Can you work these out from the model? Positions are in its coordinate system, mm. A direction names the side the tool comes from. Give positions to 0.01 mm unless a question says otherwise; leave off trailing zeros. Order: outer loops, then holes, each group sorted by start corner. A loop starts at its lowest first (then second) coordinate and runs counter-clockwise, first axis right, second up. Notation, with made-up numbers: (17, 74) - (61, 74) arc R23 cw to (61, 99) - close; hole circle Ø9 at (-33, 79). An arc over 180 degrees is marked (long way). Answer as a JSON object with one key per item and string values.
```python
from build123d import *

# Parameters (mm, degrees)
F1_DEPTH = 60
F2_SIZE  = 10
F3_SIZE2 = 70
F3_SIZE  = 40


with BuildPart() as f1:
    # F0 (on Top) → F1 (new body)
    with BuildSketch(Plane.XY):
        Polygon((0, 50), (0, 0), (10, 0), (10, 30), (90, 30), (90, 0), (110, 0), (110, 50), align=None)
    extrude(amount=F1_DEPTH)

    # F2
    f2_edges = [f1.edges().sort_by_distance(p)[0] for p in [
        (5, 0, 60),
    ]]
    chamfer(f2_edges, length=F2_SIZE)

    # F3
    f3_edges = [f1.edges().sort_by_distance(p)[0] for p in [
        (110, 25, 60),
    ]]
    f3_side = f1.faces().sort_by_distance((110, 25, 30))[0]
    chamfer(f3_edges, length=F3_SIZE, length2=F3_SIZE2, reference=f3_side)


solid = f1.part
```
Q1. If we section it at A-A, the plane y = 26.5: Please give me the cut outline in (x, z), then the cut area to 3 significant figures.
Recorded:
{"outline": "(0, 0) - (10, 0) - (10, 60) - (0, 60) - close; (90, 0) - (110, 0) - (110, 20) - (90, 31.43) - close", "area": "1,110 mm^2"}
Q2. If we section it at C-C, the plane y = 3.5: Please give me the cut outline in (x, z), then the cut area to 3 significant figures.
Recorded:
{"outline": "(0, 0) - (10, 0) - (10, 53.5) - (0, 53.5) - close; (90, 0) - (110, 0) - (110, 20) - (90, 31.43) - close", "area": "1,050 mm^2"}
Q3. We'd pull the mould along X, two halves only. Please class faces 3 (the face through (110, 25, 10)), 4 (the face through (100, 0, 12)), 5 (the face through (49, 30, 23)): released by +X, released by -X, zero draft, split by the parting line, or undercut.
Recorded:
{"face 3": "released by +X", "face 4": "zero draft", "face 5": "undercut"}
Q4. If we section it at B-B, the plane z = 11: Please give me the cut outline in (x, y).
Recorded:
{"outline": "(0, 0) - (10, 0) - (10, 30) - (90, 30) - (90, 0) - (110, 0) - (110, 50) - (0, 50) - close"}
Q5. I need wall thicknesses on L1, parallel to X at y = 9, z = 14; L2, parallel to Y at x = 16, z = 8; L3, parallel to X at y = 18, z = 29. Which ranges of each line are inside material? Lowest first, please.
Recorded:
{"L1": "x = 0 to 10, 90 to 110", "L2": "y = 30 to 50", "L3": "x = 0 to 10, 90 to 94.25"}
Q6. I'm going to push flat-ended pins straight in: pin 1 Ø6 at (y, z) = (43.5, 29) entering from +X; pin 2 Ø8 at (x, z) = (67, 17.5) entering from -Y; pin 3 Ø15 at (y, z) = (9.5, 28) entering from +X (3 decimals). Where does each tip first touch, or does it pass through?
Recorded:
{"pin 1": "stops at x = 99.5", "pin 2": "stops at y = 30", "pin 3": "stops at x = 109.125"}
Q7. If we section it at D-D, the plane x = 50.5: Please give me the cut outline in (y, z).
Recorded:
{"outline": "(30, 0) - (50, 0) - (50, 54) - (30, 54) - close"}
Q8. Which directions (+Z, -Z, +X, -X, +Y, -Y) give clear straight access to the entire face, cutting with the end or side of a thin tool? Please do faces 1 (the face through (5, 0, 25)), 2 (the face through (10, 15, 30)).
Recorded:
{"face 1": "+Z, -Z, +X, -X, -Y", "face 2": "+Z, -Z, -Y"}
